Check sheet for the modelled part. Datum: model origin and axes. Units: mm. Face numbers are marked on the shaded views. Round coordinates to 2 decimals unless told otherwise and drop trailing zeros. Write each loop counter-clockwise with the first axis right and the second up, starting at its lowest first coordinate (ties: lowest second). Pieces come first, ordered by that corner, then holes. Notation, with made-up numbers: M 27.25,51.5 L 78.25,51.5 A22 cw 78.25,85.5 Z; hole C 13,80.25 d2. An arc over 180 degrees is marked long. Answer in a Markdown table with one row per item.
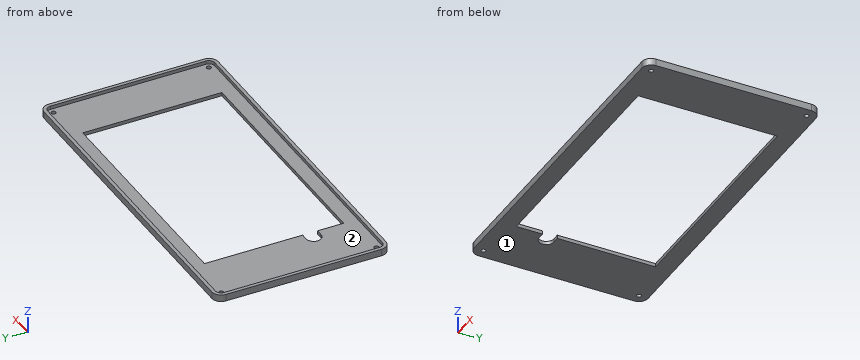
Autodesk Inventor part; units mm, degrees
ref_plane "YZ Plane" through (0, 0, 0) normal (1, 0, 0) x (0, 1, 0)
ref_plane "XZ Plane" through (0, 0, 0) normal (0, 1, 0) x (-1, 0, 0)
ref_plane "XY Plane" through (0, 0, 0) normal (0, 0, 1) x (1, 0, 0)
sketch "Sketch1" plane through (0, 0, 0) normal (0, 0, 1) x (1, 0, 0)
  line L0 (-10.4542, 14.6019) -> (210.2083, 14.6019)
  line L1 (216.5583, 8.2519) -> (216.5583, -98.1106)
  line L2 (210.2083, -104.4606) -> (-10.4542, -104.4606)
  line L3 (-16.8042, -98.1106) -> (-16.8042, 8.2519)
  line L4 (99.877, 12.2207) -> (-10.4542, 12.2207)
  line L5 (-14.423, 8.2519) -> (-14.423, -44.9293)
  line L6 (99.877, 12.2207) -> (210.2083, 12.2207)
  line L7 (214.177, 8.2519) -> (214.177, -44.9293)
  line L8 (99.877, -102.0793) -> (210.2083, -102.0793)
  line L9 (214.177, -98.1106) -> (214.177, -44.9293)
  line L10 (99.877, -102.0793) -> (-10.4542, -102.0793)
  line L11 (-14.423, -98.1106) -> (-14.423, -44.9293)
  arc A0 (-10.4542, 14.6019) -> (-16.8042, 8.2519) centre (-10.4542, 8.2519) ccw
  arc A1 (216.5583, 8.2519) -> (210.2083, 14.6019) centre (210.2083, 8.2519) ccw
  arc A2 (210.2083, -104.4606) -> (216.5583, -98.1106) centre (210.2083, -98.1106) ccw
  arc A3 (-16.8042, -98.1106) -> (-10.4542, -104.4606) centre (-10.4542, -98.1106) ccw
  arc A4 (-10.4542, 12.2207) -> (-14.423, 8.2519) centre (-10.4542, 8.2519) ccw
  arc A5 (214.177, 8.2519) -> (210.2083, 12.2207) centre (210.2083, 8.2519) ccw
  arc A6 (210.2083, -102.0793) -> (214.177, -98.1106) centre (210.2083, -98.1106) ccw
  arc A7 (-14.423, -98.1106) -> (-10.4542, -102.0793) centre (-10.4542, -98.1106) ccw
  line L12 (99.877, 2.6957) -> (22.0895, 2.6957)
  line L13 (22.0895, 2.6957) -> (22.0895, -44.9293)
  line L14 (99.877, 2.6957) -> (182.427, 2.6957)
  line L15 (182.427, 2.6957) -> (182.427, -44.9293)
  line L16 (99.877, -92.5543) -> (182.427, -92.5543)
  line L17 (182.427, -92.5543) -> (182.427, -44.9293)
  line L18 (99.877, -92.5543) -> (22.0895, -92.5543)
  line L19 (22.0895, -92.5543) -> (22.0895, -44.9293)
  point P0 (0, 0)
  point P1 (-16.8042, 14.6019)
  point P2 (216.5583, -104.4606)
  point P3 (216.5583, 14.6019)
  point P4 (-16.8042, -104.4606)
  dimension "d0" = 233.3625
  dimension "d1" = 119.0625
  dimension "d9" = 6.35
  dimension "d10" = 3.9688
  dimension "d37" = 31.75
  dimension "d38" = 36.5125
  dimension "d39" = 9.525
  dimension "d40" = 9.525
extrude "Extrusion5" add sketch "Sketch1" along normal blind 2.3813 contours L0 A1 L1 A2 L2 A3 L3 A0 | L6 A5 L7 L9 A6 L8 L10 A7 L11 L5 A4 L4
sketch "Sketch6" plane through (0, 0, 2.3813) normal (0, 0, 1) x (1, 0, 0)
  line L0 (210.2083, 14.6019) -> (-10.4542, 14.6019)
  arc A0 (-10.4542, 14.6019) -> (-16.8042, 8.2519) centre (-10.4542, 8.2519) ccw
  line L1 (-16.8042, 8.2519) -> (-16.8042, -98.1106)
  arc A1 (-16.8042, -98.1106) -> (-10.4542, -104.4606) centre (-10.4542, -98.1106) ccw
  line L2 (-10.4542, -104.4606) -> (210.2083, -104.4606)
  arc A2 (210.2083, -104.4606) -> (216.5583, -98.1106) centre (210.2083, -98.1106) ccw
  line L3 (216.5583, -98.1106) -> (216.5583, 8.2519)
  arc A3 (216.5583, 8.2519) -> (210.2083, 14.6019) centre (210.2083, 8.2519) ccw
  line L4 (99.877, 12.2207) -> (-10.4542, 12.2207)
  line L5 (-14.423, 8.2519) -> (-14.423, -44.9293)
  line L6 (99.877, 12.2207) -> (210.2083, 12.2207)
  line L7 (214.177, 8.2519) -> (214.177, -44.9293)
  line L8 (99.877, -102.0793) -> (210.2083, -102.0793)
  line L9 (214.177, -98.1106) -> (214.177, -44.9293)
  line L10 (99.877, -102.0793) -> (-10.4542, -102.0793)
  line L11 (-14.423, -98.1106) -> (-14.423, -44.9293)
  arc A4 (-10.4542, 12.2207) -> (-14.423, 8.2519) centre (-10.4542, 8.2519) ccw
  arc A5 (214.177, 8.2519) -> (210.2083, 12.2207) centre (210.2083, 8.2519) ccw
  arc A6 (210.2083, -102.0793) -> (214.177, -98.1106) centre (210.2083, -98.1106) ccw
  arc A7 (-14.423, -98.1106) -> (-10.4542, -102.0793) centre (-10.4542, -98.1106) ccw
  point P0 (0, 0)
  dimension "d47" = 3.9688
extrude "Extrusion6" add sketch "Sketch6" along normal blind 2.3813
sketch "Sketch12" plane through (0, 0, 0) normal (0, 0, -1) x (-1, 0, 0)
  arc A0 (-210.2083, 14.6019) -> (-216.5583, 8.2519) centre (-210.2083, 8.2519) ccw
  arc A1 (-216.5583, -98.1106) -> (-210.2083, -104.4606) centre (-210.2083, -98.1106) ccw
  arc A2 (10.4542, -104.4606) -> (16.8042, -98.1106) centre (10.4542, -98.1106) ccw
  arc A3 (16.8042, 8.2519) -> (10.4542, 14.6019) centre (10.4542, 8.2519) ccw
  circle A4 centre (10.4542, 8.2519) radius 1.5875
  circle A5 centre (10.4542, -98.1106) radius 1.5875
  circle A6 centre (-210.2083, -98.1106) radius 1.5875
  circle A7 centre (-210.2083, 8.2519) radius 1.5875
  point P0 (0, 0)
  dimension "d64" = 3.175
  dimension "d65" = 3.175
  dimension "d66" = 3.175
  dimension "d67" = 3.175
hole "Hole2" at (210.2083, 8.2519, 0) at (-10.4542, 8.2519, 0) at (-10.4542, -98.1106, 0) at (210.2083, -98.1106, 0) direction (0, 0, 1) diameter 3.175 end through all
sketch "Sketch13" plane through (0, 0, 0) normal (0, 0, -1) x (-1, 0, 0)
  line L0 (-22.0895, 2.6957) -> (-22.0895, -92.5543)
  line L1 (16.8042, -98.1106) -> (16.8042, 8.2519)
  line L2 (16.8042, -89.9075) -> (-17.435, -89.9075)
  arc A0 (-17.435, -74.641) -> (-17.435, -64.481) centre (-17.435, -69.561) ccw
  line L3 (-17.435, -64.481) -> (-22.0895, -64.481)
  line L4 (-17.435, -74.641) -> (-22.0895, -74.641)
  line L5 (-22.0895, -64.481) -> (-22.0895, -74.641)
  point P0 (0, 0)
  dimension "d75" = 34.2392
split body "Split3" sketch "Sketch13" result one side removed curves L3 L5 L4 A0 removed pieces at (20.538, -71.2543, 0.5)
properties part number "Slave Tablet Cover"
1. Section check B-B, the plane x = 140.5. Record the cut outline in (y, z).
Found:
| item | result |
|---|---|
| outline | M -104.46,0 L -92.55,0 L -92.55,2.38 L -102.08,2.38 L -102.08,4.76 L -104.46,4.76 Z; M 2.7,0 L 14.6,0 L 14.6,4.76 L 12.22,4.76 L 12.22,2.38 L 2.7,2.38 Z |
2. Scan lines: L1, parallel to X at y = -22, z = 1.05; L2, parallel to X at y = -61.5, z = 3.95; L3, parallel to Y at x = 33, z = 2.6. Record each from-to range of solid material in increasing order.
Found:
| item | result |
|---|---|
| L1 | x = -16.8 to 22.09, 182.43 to 216.56 |
| L2 | x = -16.8 to -14.42, 214.18 to 216.56 |
| L3 | y = -104.46 to -102.08, 12.22 to 14.6 |
3. Section check C-C, the plane z = 1. Count the separate pieces of the cut face and the enclosed holes in it, and give its area (3 significant figures).
Found:
| item | result |
|---|---|
| separate pieces | 1 |
| enclosed holes | 5 |
| area | 12,400 mm2 |
4. Go/stop test with flat-tipped pins: pin 1 (2.5 mm diameter, centred on x = 210.21, y = 8.25, fed in from +Z); pin 2 (2 mm diameter, centred on x = 16, y = -74, fed in from +Z). Record where each tip stops, or that it passes through.
Found:
| item | result |
|---|---|
| pin 1 | passes through |
| pin 2 | stops at z = 2.38 |
5. Section check A-A, the plane y = -90. Record the cut outline in (x, z).
Found:
| item | result |
|---|---|
| outline | M -16.8,0 L 22.09,0 L 22.09,2.38 L -14.42,2.38 L -14.42,4.76 L -16.8,4.76 Z; M 182.43,0 L 216.56,0 L 216.56,4.76 L 214.18,4.76 L 214.18,2.38 L 182.43,2.38 Z |
6. Draft check along X on the marked faces 1 and 2. Enter one of: +X half, -X half, draft (parallel to the pull), parting line (faces both ways), or undercut.
Found:
| item | result |
|---|---|
| face 1 | draft |
| face 2 | undercut |
